```python
from build123d import *

# Parameters (mm, degrees)
BASE_FLANGE1_DEPTH = 40
SKETCH6_R          = 2
CUT_EXTRUDE1_DEPTH = 10
SKETCH7_R          = 5
SKETCH7_R_2        = 1.75
CUT_EXTRUDE2_DEPTH = 10
SKETCH8_R          = 1.6
CUT_EXTRUDE3_DEPTH = 10
EDGE_FLANGE1_DEPTH = 100
FILLET1_R          = 5
SKETCH12_W         = 12
SKETCH12_H         = 12
CUT_EXTRUDE4_DEPTH = 10


# Sheet-metal steps are written as plain solids
with BuildPart() as part:
    # Sketch1 → Base-Flange1 (new body)
    with BuildSketch(Plane.XY):
        with BuildLine():
            Line((0, 0), (0, 46))
            ThreePointArc((0, 46), (1.171572875, 48.828427125), (4, 50))
            Line((4, 50), (175, 50))
            Line((175, 50), (175, 48))
            Line((175, 48), (4, 48))
            ThreePointArc((4, 48), (2.585786438, 47.414213562), (2, 46))
            Line((2, 46), (2, 0))
            Line((2, 0), (0, 0))
        make_face()
    extrude(amount=BASE_FLANGE1_DEPTH)

    # Sketch6 → Cut-Extrude1 (cut)
    with BuildSketch(Plane.ZY):
        with Locations((5, 41)):
            Circle(SKETCH6_R)
        with Locations((35, 5)):
            Circle(SKETCH6_R)
    extrude(amount=-CUT_EXTRUDE1_DEPTH, mode=Mode.SUBTRACT)

    # Sketch7 → Cut-Extrude2 (cut)
    with BuildSketch(Plane(origin=(0, 50, 0), x_dir=(1, 0, 0), z_dir=(0, 1, 0))):
        with Locations(Location((150, -20, 0), (0, 0, 270))):
            Circle(SKETCH7_R)
        with Locations(Location((132.5, -28, 0), (0, 0, 270))):
            Circle(SKETCH7_R_2)
        with Locations(Location((167.5, -28, 0), (0, 0, 270))):
            Circle(SKETCH7_R_2)
    extrude(amount=-CUT_EXTRUDE2_DEPTH, mode=Mode.SUBTRACT)

    # Sketch8 → Cut-Extrude3 (cut)
    with BuildSketch(Plane(origin=(0, 50, 0), x_dir=(1, 0, 0), z_dir=(0, 1, 0))):
        with Locations(Location((20.208399829, -9.85, 0), (0, 0, 270))):
            Circle(SKETCH8_R)
        with Locations(Location((63.408399829, -9.85, 0), (0, 0, 270))):
            Circle(SKETCH8_R)
        with Locations(Location((63.408399829, -30.15, 0), (0, 0, 270))):
            Circle(SKETCH8_R)
        with Locations(Location((20.208399829, -30.15, 0), (0, 0, 270))):
            Circle(SKETCH8_R)
    extrude(amount=-CUT_EXTRUDE3_DEPTH, mode=Mode.SUBTRACT)

    # Edge-Flange1 section (across the edge) → Edge-Flange1 (add)
    with BuildSketch(Plane(origin=(104, 48, 42), x_dir=(0, 0, -1), z_dir=(-1, 0, 0))):
        with BuildLine():
            Line((-2, 2), (-2, 33))
            Line((-2, 33), (0, 33))
            Line((0, 33), (0, 2))
            ThreePointArc((0, 2), (0.585786438, 0.585786438), (2, 0))
            Line((2, 0), (2, -2))
            ThreePointArc((2, -2), (-0.828427125, -0.828427125), (-2, 2))
        make_face()
    extrude(amount=EDGE_FLANGE1_DEPTH)

    # Fillet1
    fillet1_edges = [part.edges().sort_by_distance(p)[0] for p in [
        (104, 15, 43),
        (4, 15, 43),
        (1, 0, 40),
        (175, 49, 40),
        (1, 0, 0),
        (175, 49, 0),
    ]]
    fillet(fillet1_edges, radius=FILLET1_R)

    # Sketch12 → Cut-Extrude4 (cut)
    with BuildSketch(Plane.XY.offset(44)):
        with Locations((20, 31)):
            Rectangle(SKETCH12_W, SKETCH12_H)
        with Locations((35, 31)):
            Rectangle(SKETCH12_W, SKETCH12_H)
        with Locations((50, 31)):
            Rectangle(SKETCH12_W, SKETCH12_H)
        with Locations((65, 31)):
            Rectangle(SKETCH12_W, SKETCH12_H)
    extrude(amount=-CUT_EXTRUDE4_DEPTH, mode=Mode.SUBTRACT)


solid = part.part
```
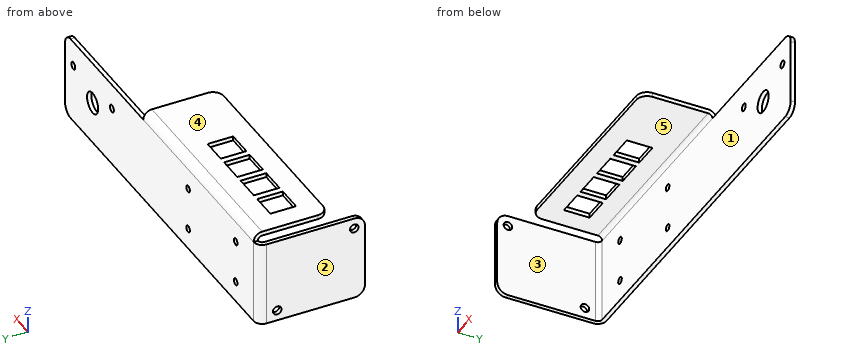
The listing builds one solid part. Answer for the finished solid, in the listing's coordinates (mm). Face numbers are marked on the shaded views. A direction names the side the tool comes from. Coordinates: 2 decimals unless noted, no trailing zeros. Order: outer loops, then holes, each group sorted by start corner. A loop starts at its lowest first (then second) coordinate and runs counter-clockwise, first axis right, second up. Notation, with made-up numbers: M 82,34.25 L 141,34.25 A17 ccw 141,46.25 Z; hole C 31.25,57 d11. An arc over 180 degrees is marked long. Answer as a JSON object with one key per item and string values. Group by question number.
1. Flat-ended cylindrical pins translate along their axes: P1, Ø1.6, axis at x = 33.5, z = 43, coming from the -Y side; P2, Ø3, axis at x = 42.5, z = 31.5, coming from the -Y side; P3, Ø1.2, axis at y = 32.5, z = 42, coming from the -X side; P4, Ø2, axis at y = 31.5, z = 5, coming from the -X side. Find the tip coordinate at first contact, or state that the pin passes through.
2. Section C-C on y = 41 is taken. Write down the section's boundary in (x, z), then the cut area to 3 significant figures.
3. Section B-B on z = 9.85 is taken. Write down the section's boundary in (x, y), then the cut area to 3 significant figures.
4. Straight lines are drawn through the part: line 1 (X direction, y = 49.55, z = 9.85); line 2 (Y direction, x = 0.55, z = 5); line 3 (X direction, y = 38.5, z = 34). For each, find the intervals that lie inside material, in ascending order.
5. Section D-D on z = 18 is taken. Write down the section's boundary in (x, y).
6. A tool of negligible diameter and unlimited length cuts with its end or side. For the marked faces 1, 2, 3, 4 and 5, from which of +Z, -Z, +X, -X, +Y, -Y can it reach the whole face along a straight path? Write none if from no direction.
7. Section A-A on x = 132.5 is taken. Write down the section's boundary in (y, z).
Values follow:
{
 "1": {"P1": "y = 15", "P2": "y = 48", "P3": "x = 4", "P4": "x = 0"},
 "2": {"outline": "M 0,0 L 2,0 L 2,3 L 0,3 Z; M 0,7 L 2,7 L 2,40 L 0,40 Z; M 4,42 L 104,42 L 104,44 L 4,44 Z", "area": "272 mm2"},
 "3": {"outline": "M 0,0 L 2,0 L 2,46 A2 cw 4,48 L 18.61,48 L 18.61,50 L 4,50 A4 ccw 0,46 Z; M 21.81,48 L 61.81,48 L 61.81,50 L 21.81,50 Z; M 65.01,48 L 175,48 L 175,50 L 65.01,50 Z", "area": "431 mm2"},
 "4": {"line 1": "2.16 to 18.61, 21.81 to 61.81, 65.01 to 175", "line 2": "0 to 39, 43 to 48.02", "line 3": "0 to 2"},
 "5": {"outline": "M 0,0 L 2,0 L 2,46 A2 cw 4,48 L 145.42,48 L 145.42,50 L 4,50 A4 ccw 0,46 Z; M 154.58,48 L 175,48 L 175,50 L 154.58,50 Z"},
 "6": {"face 1": "-Z, +X, -Y", "face 2": "+Z, -Z, -X, +Y, -Y", "face 3": "+Z, -Z, +X, -Y", "face 4": "+Z, +X, -X, +Y, -Y", "face 5": "-Z, +X, -X, -Y"},
 "7": {"outline": "M 48,0 L 50,0 L 50,26.25 L 48,26.25 Z; M 48,29.75 L 50,29.75 L 50,40 L 48,40 Z"}
}
